CAD build for the part. Positions are in the model's coordinates, mm. Face numbers are marked on the shaded views. Give positions to 0.01 mm unless a question says otherwise; leave off trailing zeros. Write each loop counter-clockwise with the first axis right and the second up, starting at its lowest first coordinate (ties: lowest second). Pieces come first, ordered by that corner, then holes. Notation, with made-up numbers: (24, 89.5) -> (76, 89.5) arc R19 cw to (76, 109.5) -> close; hole circle Ø8 at (40, 45.5). An arc over 180 degrees is marked (long way). Answer as a JSON object with one key per item and string values.
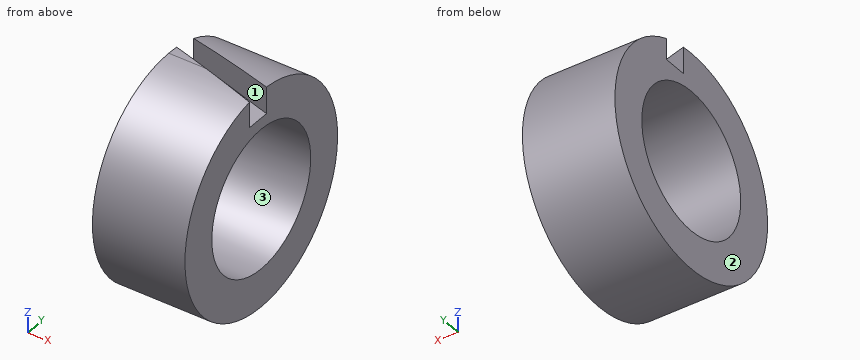
```python
from build123d import *

# Parameters (mm, degrees)
F0_W     = 67.935511
F0_H     = 28.069519
F4_DEPTH = 20.973967


with BuildPart() as f1:
    # F0 (on Front) → F1 (revolve)
    with BuildSketch(Plane.XZ):
        with Locations((1.417562, 38.79952)):
            Rectangle(F0_W, F0_H)
    revolve(axis=Axis((8.571956, 0, -26.890948), (1, 0, 0)))

    # F3 (on offset) → F4 (cut)
    with BuildSketch(Plane.XY.offset(53.962)):
        Polygon((53.347535, 0), (-46.056576, 30.157462), (-45.957059, 12.388781), (53.227343, -17.801717), align=None)
    extrude(amount=-F4_DEPTH, mode=Mode.SUBTRACT)


solid = f1.part
```
1) Wall check: probe 1 along Z at (x, y) = (9, 0); probe 2 along Y at (x, z) = (-24, -28); probe 3 along Z at (x, y) = (-6, 0). Give the ranges that are in metal, low to high.
Model answer:
{"probe 1": "z = -106.62 to -78.55, 24.76 to 32.99", "probe 2": "y = -79.72 to -51.64, 51.64 to 79.72", "probe 3": "z = -106.62 to -78.55, 24.76 to 52.83"}
2) Slice it at A-A (z = -16.5). List the corners of the cut face in (x, y), then the cut area to 3 significant figures.
Model answer:
{"outline": "(-32.55, -79.05) -> (35.39, -79.05) -> (35.39, -50.6) -> (-32.55, -50.6) -> close; (-32.55, 50.6) -> (35.39, 50.6) -> (35.39, 79.05) -> (-32.55, 79.05) -> close", "area": "3,860 mm2"}
3) Slice it at D-D (z = -48). List the corners of the cut face in (x, y), then the cut area to 3 significant figures.
Model answer:
{"outline": "(-32.55, -76.88) -> (35.39, -76.88) -> (35.39, -47.15) -> (-32.55, -47.15) -> close; (-32.55, 47.15) -> (35.39, 47.15) -> (35.39, 76.88) -> (-32.55, 76.88) -> close", "area": "4,040 mm2"}
4) Pin check, flat tips, straight feed: pin 1 (10 mm diameter, centred on x = 3, z = 0, fed in from +Y); pin 2 (12 mm diameter, centred on x = 21.5, z = -19, fed in from +Y); pin 3 (2 mm diameter, centred on x = 27.5, y = -31.5, fed in from +Z). Stop position of each tip, or through.
Model answer:
{"pin 1": "stops at y = 76.66", "pin 2": "stops at y = 79.7", "pin 3": "stops at z = 46.77"}
5) Mould opens along Y. For the marked faces 1, 2 and 3 say: released by +Y, released by -Y, zero draft, split by the parting line, or undercut.
Model answer:
{"face 1": "undercut", "face 2": "zero draft", "face 3": "undercut"}
6) Slice it at B-B (y = 15.5). List the corners of the cut face in (x, z), then the cut area to 3 significant figures.
Model answer:
{"outline": "(-32.55, -105.09) -> (35.39, -105.09) -> (35.39, -76.17) -> (-32.55, -76.17) -> close; (-32.55, 22.38) -> (35.39, 22.38) -> (35.39, 51.31) -> (2.26, 51.31) -> (2.26, 32.99) -> (-32.55, 32.99) -> close", "area": "3,290 mm2"}
7) Slice it at C-C (x = -18.5). List the corners of the cut face in (y, z).
Model answer:
{"outline": "(4.03, 32.99) -> (4.03, 52.73) arc R79.73 ccw (long way) to (21.8, 49.8) -> (21.8, 32.99) -> close; hole circle Ø103.31 at (0, -26.89)"}
